The listing builds one solid part. Answer for the finished solid, in the listing's coordinates (mm). Face numbers are marked on the shaded views. Round coordinates to 2 decimals unless told otherwise and drop trailing zeros. Loops run counter-clockwise (first coordinate to the right, second up) from the corner with the lowest first, then second, coordinate; pieces in that order, holes last. Notation, with made-up numbers: (31, 63) -> (48, 63) arc R26 ccw to (48, 77) -> close; hole circle Ø3 at (63, -10.5). An arc over 180 degrees is marked (long way). One line per question, with ' | ' between items.
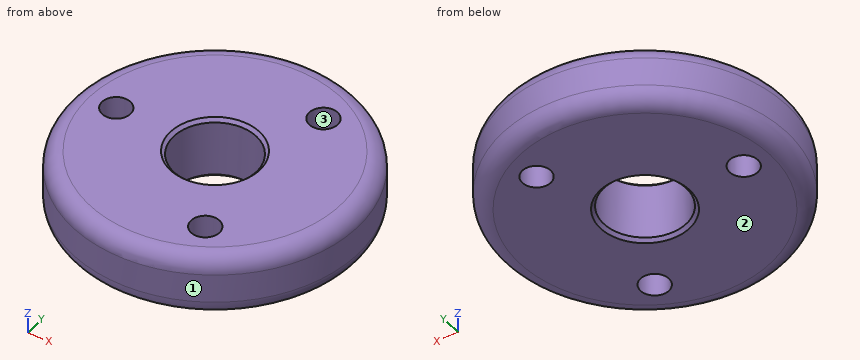
from build123d import *

# Parameters (mm, degrees)
SKETCH1_R           = 5.461
SKETCH1_R_2         = 1.5875
BOSS_EXTRUDE1_DEPTH = 1.190625
FILLET1_R           = 0.635
CHAMFER1_SIZE       = 0.127
SKETCH2_R           = 0.5461
CUT_EXTRUDE1_DEPTH  = 9.081794025
CIRPATTERN1_COUNT   = 3


with BuildPart() as part:
    # Sketch1 → Boss-Extrude1 (new, symmetric)
    with BuildSketch(Plane.XY):
        with Locations(Location((0, 0, 0), (0, 0, 180))):
            Circle(SKETCH1_R)
        with Locations(Location((0, 0, 0), (0, 0, 180))):
            Circle(SKETCH1_R_2, mode=Mode.SUBTRACT)
    extrude(amount=BOSS_EXTRUDE1_DEPTH, both=True)

    # Fillet1
    fillet1_edges = [part.edges().sort_by_distance(p)[0] for p in [
        (5.461, 0, -1.190625),
        (5.461, 0, 1.190625),
    ]]
    fillet(fillet1_edges, radius=FILLET1_R)

    # Chamfer1
    chamfer1_edges = [part.edges().sort_by_distance(p)[0] for p in [
        (1.5875, 0, -1.190625),
        (1.5875, 0, 1.190625),
    ]]
    chamfer(chamfer1_edges, length=CHAMFER1_SIZE)

    # Sketch2 → Cut-Extrude1 (cut, through all)
    with BuildSketch(Plane.XY.offset(1.190625)):
        with Locations((-3.81, 0)):
            Circle(SKETCH2_R)
    cut_extrude1 = extrude(amount=-CUT_EXTRUDE1_DEPTH, mode=Mode.SUBTRACT)

    # CirPattern1: Cut-Extrude1 ×3 about axis
    cirpattern1_axis = Axis((0, 0, 0), (0, 0, 1))
    for i in range(1, CIRPATTERN1_COUNT):
        add(cut_extrude1.rotate(cirpattern1_axis, i * 360 / CIRPATTERN1_COUNT), mode=Mode.SUBTRACT)


solid = part.part
Q1. A cutting plane is placed at B-B on y = 0. Give the number of separate pieces and of enclosed holes in the cut face, plus the area to 3 significant figures.
Numbers:
separate pieces: 3 | enclosed holes: 0 | area: 15.5 mm^2
Q2. Given pin 1 Ø1.9 at (x, y) = (0, 0) entering from -Z (3 decimals), flat-ended and moving along its own axis, determine where the tip first touches the part or whether it passes through.
Numbers:
pin 1: through
Q3. A cutting plane is placed at C-C on z = -0.3. Give the vertices of the cut face in (x, y) (1 decimal).
Numbers:
outline: circle Ø10.9 at (0, 0); hole circle Ø1.1 at (-3.8, 0); hole circle Ø3.2 at (0, 0); hole circle Ø1.1 at (1.9, -3.3); hole circle Ø1.1 at (1.9, 3.3)
Q4. For a pull along Y with two mould halves and no side action, classify the marked faces 1, 2 and 3 as pulls with the +Y half, pulls with the -Y half, needs draft (parallel to the pull), parting line crosses it, or undercut.
Numbers:
face 1: parting line crosses it | face 2: needs draft | face 3: undercut
Q5. Find the intervals of material crossed by line 1 (X direction, y = -0.25, z = 0.5); line 2 (Y direction, x = 2.25, z = -0.05); line 3 (Y direction, x = 1.75, z = 0.3), in increasing order. Write a range as from..to.
Numbers:
line 1: -5.46..-4.3, -3.32..-1.57, 1.57..5.46 | line 2: -4.98..-3.72, -2.88..2.88, 3.72..4.98 | line 3: -5.17..-3.82, -2.78..2.78, 3.82..5.17
